Check sheet for the modelled part. Datum: model origin and axes. Units: mm. Face numbers are marked on the shaded views. Give positions to 0.01 mm unless a question says otherwise; leave off trailing zeros. Write each loop counter-clockwise with the first axis right and the second up, starting at its lowest first coordinate (ties: lowest second). Pieces come first, ordered by that corner, then holes. Notation, with made-up numbers: M 66.25,9.5 L 70.25,9.5 A32 cw 70.25,43.5 Z; hole C 6,42.5 d4. An arc over 180 degrees is marked long. One line per item, written item: value. Start each with the question number.
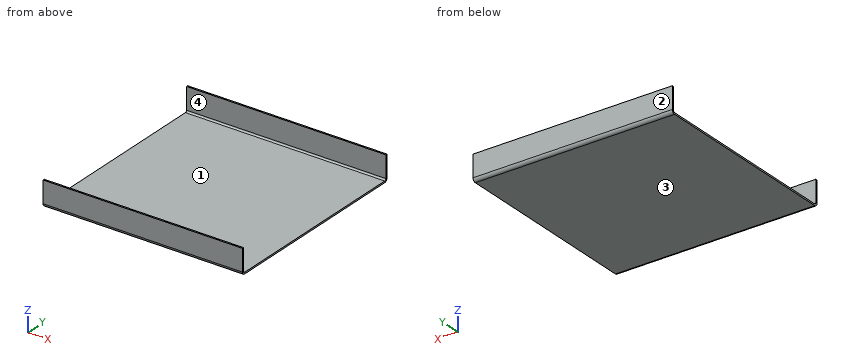
from build123d import *

# Parameters (mm, degrees)
SKETCH1_W                      = 203.2
SKETCH1_H                      = 203.2
BOSS_EXTRUDE2_DEPTH            = 1.5875
EDGE_FLANGE1_STRIP_W           = 9.525
EDGE_FLANGE1_STRIP_H           = 1.5875
EDGE_FLANGE1_STRIP_CUT_DEPTH   = 203.2
EDGE_FLANGE1_STRIP_2_W         = 9.525
EDGE_FLANGE1_STRIP_2_H         = 1.5875
EDGE_FLANGE1_STRIP_CUT_2_DEPTH = 203.2
EDGE_FLANGE1_DEPTH             = 203.2
EDGE_FLANGE1_BEND_DEPTH        = 203.2


# Sheet-metal steps are written as plain solids
with BuildPart() as part:
    # Sketch1 → Boss-Extrude2 (new body)
    with BuildSketch(Plane.XY):
        with Locations((101.6, 101.6)):
            Rectangle(SKETCH1_W, SKETCH1_H)
    extrude(amount=BOSS_EXTRUDE2_DEPTH)

    # Edge-Flange1 strip (across the edge) → Edge-Flange1 strip cut (cut)
    with BuildSketch(Plane(origin=(203.2, 203.2, 1.5875), x_dir=(0, -1, 0), z_dir=(-1, 0, 0))):
        with Locations((-1.5875, -0.79375)):
            Rectangle(EDGE_FLANGE1_STRIP_W, EDGE_FLANGE1_STRIP_H)
    extrude(amount=EDGE_FLANGE1_STRIP_CUT_DEPTH, mode=Mode.SUBTRACT)

    # Edge-Flange1 strip 2 (across the edge) → Edge-Flange1 strip cut 2 (cut)
    with BuildSketch(Plane(origin=(0, 0, 1.5875), x_dir=(0, 1, 0), z_dir=(1, 0, 0))):
        with Locations((-1.5875, -0.79375)):
            Rectangle(EDGE_FLANGE1_STRIP_2_W, EDGE_FLANGE1_STRIP_2_H)
    extrude(amount=EDGE_FLANGE1_STRIP_CUT_2_DEPTH, mode=Mode.SUBTRACT)

    # Edge-Flange1 section (across the edge) → Edge-Flange1 (add)
    with BuildSketch(Plane(origin=(203.2, 203.2, 1.5875), x_dir=(0, -1, 0), z_dir=(-1, 0, 0))):
        with BuildLine():
            Line((0, 1.5875), (0, 23.8125))
            Line((0, 23.8125), (1.5875, 23.8125))
            Line((1.5875, 23.8125), (1.5875, 1.5875))
            ThreePointArc((1.5875, 1.5875), (2.052467985, 0.464967985), (3.175, 0))
            Line((3.175, 0), (3.175, -1.5875))
            ThreePointArc((3.175, -1.5875), (0.92993597, -0.65756403), (0, 1.5875))
        make_face()
    extrude(amount=EDGE_FLANGE1_DEPTH)

    # Edge-Flange1 section 2 (across the edge) → Edge-Flange1 bend (add)
    with BuildSketch(Plane(origin=(0, 0, 1.5875), x_dir=(0, 1, 0), z_dir=(1, 0, 0))):
        with BuildLine():
            Line((0, 1.5875), (0, 23.8125))
            Line((0, 23.8125), (1.5875, 23.8125))
            Line((1.5875, 23.8125), (1.5875, 1.5875))
            ThreePointArc((1.5875, 1.5875), (2.052467985, 0.464967985), (3.175, 0))
            Line((3.175, 0), (3.175, -1.5875))
            ThreePointArc((3.175, -1.5875), (0.92993597, -0.65756403), (0, 1.5875))
        make_face()
    extrude(amount=EDGE_FLANGE1_BEND_DEPTH)


solid = part.part
1) Cross-section at A-A (z = 22). Record the boundary of the cut face in (x, y).
2) Cross-section at C-C (y = 74). Record the boundary of the cut face in (x, z), plus the area to 3 significant figures.
3) Material ranges on L1, parallel to Y at x = 175.5, z = 15.5; L2, parallel to Z at x = 88.5, y = 128; L3, parallel to Y at x = 184.5, z = 2.25, recorded low to high. Write a range as from..to.
4) Draft check along Y on the marked faces 1, 2, 3 and 4. Enter one of: released by +Y, released by -Y, zero draft, split by the parting line, or undercut.
5) Gauge pin test, flat end, axial feed: pin 1 (2 mm diameter, centred on x = 39, y = 68.5, fed in from +Z). Record the tip position at first contact, or that the pin passes through.
Data:
1. outline: M 0,0 L 203.2,0 L 203.2,1.59 L 0,1.59 Z; M 0,201.61 L 203.2,201.61 L 203.2,203.2 L 0,203.2 Z
2. outline: M 0,0 L 203.2,0 L 203.2,1.59 L 0,1.59 Z
2. area: 323 mm2
3. L1: y = 0..1.59, 201.61..203.2
3. L2: z = 0..1.59
3. L3: y = 0.14..1.88, 201.32..203.06
4. face 1: undercut
4. face 2: released by +Y
4. face 3: zero draft
4. face 4: undercut
5. pin 1: stops at z = 1.59
